from build123d import *

# Parameters (mm, degrees)
CHANFREIN1_SIZE = 1


with BuildPart() as part:
    # Esquisse1 → Révolution1 (revolve)
    with BuildSketch(Plane.XY, mode=Mode.PRIVATE) as r_volution1_sk:
        Polygon((-39, 0), (-39, 7.95), (-25, 7.95), (-25, 10.95), (25, 10.95), (25, 7.95), (39, 7.95), (39, 0), align=None)
    revolve(r_volution1_sk.sketch.rotate(Axis((-49.116366612, 0, 0), (1, 0, 0)), 180), axis=Axis((-49.116366612, 0, 0), (1, 0, 0)))

    # Chanfrein1
    chanfrein1_edges = [part.edges().sort_by_distance(p)[0] for p in [
        (39, 7.95, 0),
        (25, 10.95, 0),
        (-25, 10.95, 0),
        (-39, 7.95, 0),
    ]]
    chamfer(chanfrein1_edges, length=CHANFREIN1_SIZE)


solid = part.part
The listing builds one solid part. Answer for the finished solid, in the listing's coordinates (mm). A direction names the side the tool comes from. Coordinates: 2 decimals unless noted, no trailing zeros. Write each loop counter-clockwise with the first axis right and the second up, starting at its lowest first coordinate (ties: lowest second). Pieces come first, ordered by that corner, then holes. Notation, with made-up numbers: M 23.25,41 L 56.25,41 A16 ccw 56.25,68 Z; hole C 42.5,-20 d2. An arc over 180 degrees is marked long. Use one line per item in the form item = value.
Item 1: Find section B-B, the plane x = 19.5. Give the vertices of the cut face in (y, z).
Model answer:
outline = C 0,0 d21.9
Item 2: Find the intervals of material crossed by probe 1 along Z at (x, y) = (2.5, -0.5); probe 2 along Z at (x, y) = (-28, 0.5); probe 3 along Y at (x, z) = (11.5, -1.25), in increasing order.
Model answer:
probe_1 = -10.94 to 10.94
probe_2 = -7.93 to 7.93
probe_3 = -10.88 to 10.88
Item 3: For faces 1 (the face through (-25, -0.8, 8.1)), 2 (the face through (25, 0.8, 8.1)), 3 (the face through (39, 0, 0)), determine the directions among +Z, -Z, +X, -X, +Y, -Y from which every point of the face is accessible in a straight line to the end or side of a thin tool.
Model answer:
face_1 = -X
face_2 = +X
face_3 = +Z, -Z, +X, +Y, -Y
Item 4: Find section A-A, the plane y = 0. Give the vertices of the cut face in (x, z).
Model answer:
outline = M -39,-6.95 L -38,-7.95 L -25,-7.95 L -25,-9.95 L -24,-10.95 L 24,-10.95 L 25,-9.95 L 25,-7.95 L 38,-7.95 L 39,-6.95 L 39,6.95 L 38,7.95 L 25,7.95 L 25,9.95 L 24,10.95 L -24,10.95 L -25,9.95 L -25,7.95 L -38,7.95 L -39,6.95 Z
Item 5: Given P1, Ø8, axis at x = -15, z = -8, coming from the +Y side; P2, Ø1.5, axis at y = 3.5, z = -8.5, coming from the +X side; P3, Ø2, axis at x = -29, y = -7, coming from the +Z side, each flat-ended and moving along its own axis, determine where each tip first touches the part or whether it passes through.
Model answer:
P1 = 10.19
P2 = 25
P3 = 5.22
Item 6: Find section C-C, the plane x = 28.5. Give the vertices of the cut face in (y, z).
Model answer:
outline = C 0,0 d15.9
